```python
from build123d import *

# Parameters (mm, degrees)
BASE_W                                          = 50
BASE_H                                          = 26
BOSS_EXTRUDE2_DEPTH                             = 3
SKETCH2_R                                       = 6.35
BOSS_EXTRUDE1_DEPTH                             = 20
SKETCH7_R                                       = 4.7625
CUT_EXTRUDE1_DEPTH                              = 15
BOSS_EXTRUDE8_REACH                             = 47.531
CSK_FOR_M5_FLAT_HEAD_MACHINE_SCREW2_D           = 5.3
CSK_FOR_M5_FLAT_HEAD_MACHINE_SCREW2_DEPTH       = 10
CSK_FOR_M5_FLAT_HEAD_MACHINE_SCREW2_CSINK_D     = 10.4
CSK_FOR_M5_FLAT_HEAD_MACHINE_SCREW2_CSINK_ANGLE = 90
CSK_FOR_M5_FLAT_HEAD_MACHINE_SCREW2_TIP         = 1.59228064


with BuildPart() as part:
    # Base → Boss-Extrude2 (new body)
    with BuildSketch(Plane.XY):
        Rectangle(BASE_W, BASE_H)
    extrude(amount=BOSS_EXTRUDE2_DEPTH)

    # Sketch6 → Loft2 section 0
    with BuildSketch(Plane.XY.offset(23)):
        with BuildLine():
            Line((-5, 13), (5, 13))
            Line((5, 13), (5, 6.65))
            Line((5, 6.65), (-5, 6.65))
            Line((-5, 6.65), (-5, 13))
        make_face()
    # Sketch5 → Loft2 section 1
    with BuildSketch(Plane.XY.offset(3)):
        with BuildLine():
            Line((-25, 13), (25, 13))
            Line((25, 13), (25, 6.65))
            Line((25, 6.65), (-25, 6.65))
            Line((-25, 6.65), (-25, 13))
        make_face()
    loft()



with BuildPart() as body_2:
    # Sketch2 → Boss-Extrude1 (new body)
    with BuildSketch(Plane(origin=(-16.995934691, 0, 52.308108396), x_dir=(0.9510565162951523, 0, 0.3090169943749514), z_dir=(-0.3090169943749514, 0, 0.9510565162951523))):
        with Locations((11.371412907, 9.08)):
            Circle(SKETCH2_R)
    extrude(amount=-BOSS_EXTRUDE1_DEPTH)

    # Sketch7 → Cut-Extrude1 (cut)
    with BuildSketch(Plane(origin=(-16.995934691, 0, 52.308108396), x_dir=(0.9510565162951523, 0, 0.3090169943749514), z_dir=(-0.3090169943749514, 0, 0.9510565162951523))):
        with Locations((11.371412907, 9.08)):
            Circle(SKETCH7_R)
    extrude(amount=-CUT_EXTRUDE1_DEPTH, mode=Mode.SUBTRACT)


with BuildPart() as part_1:
    add(part.part)

    add(body_2.part)  # Boss-Extrude8 merges body 2
    # Boss-Extrude8: up to this plane
    boss_extrude8_end = Plane(origin=(-0.000738458, 9.08, 36.800937909), z_dir=(-0.3090169943749514, 0, 0.9510565162951523))
    # Sketch17 → Boss-Extrude8 (add, up to the surface)
    with BuildSketch(Plane.XY.offset(23), mode=Mode.PRIVATE) as boss_extrude8_sk1:
        Polygon((-4.751504294, 13.000455244), (-4.751504294, 6.647086382), (4.750367151, 6.647086382), (4.750367151, 13), align=None)
    boss_extrude8_tool1 = split(extrude(boss_extrude8_sk1.sketch, amount=BOSS_EXTRUDE8_REACH, mode=Mode.PRIVATE), bisect_by=boss_extrude8_end, keep=Keep.BOTH, mode=Mode.PRIVATE)
    add(boss_extrude8_tool1.solids().sort_by_distance((-0.000625, 9.823657, 23))[0])

    # CSK for M5 Flat Head Machine Screw2
    with Locations(Plane.XY.offset(3)):
        with Locations((-15, -1.5), (15, -1.5)):
            CounterSinkHole(CSK_FOR_M5_FLAT_HEAD_MACHINE_SCREW2_D / 2, CSK_FOR_M5_FLAT_HEAD_MACHINE_SCREW2_CSINK_D / 2, depth=CSK_FOR_M5_FLAT_HEAD_MACHINE_SCREW2_DEPTH, counter_sink_angle=CSK_FOR_M5_FLAT_HEAD_MACHINE_SCREW2_CSINK_ANGLE)
            with Locations((0, 0, -(CSK_FOR_M5_FLAT_HEAD_MACHINE_SCREW2_DEPTH + CSK_FOR_M5_FLAT_HEAD_MACHINE_SCREW2_TIP / 2))):  # 118° drill point
                Cone(0, CSK_FOR_M5_FLAT_HEAD_MACHINE_SCREW2_D / 2, CSK_FOR_M5_FLAT_HEAD_MACHINE_SCREW2_TIP, mode=Mode.SUBTRACT)


solid = part_1.part
```
Input: part model. Units: mm. Frame: model coordinates. A direction names the side the tool comes from. Coordinates: 2 decimals unless noted, no trailing zeros. Loops run counter-clockwise (first coordinate to the right, second up) from the corner with the lowest first, then second, coordinate; pieces in that order, holes last. Notation, with made-up numbers: M -37,63 L -20,63 A24 cw -20,100 Z; hole C 25,29.5 d3. An arc over 180 degrees is marked long. Use a Markdown table: item, result. Add a question column.
1) Pin query (flat end, axial travel): P1, Ø8, axis at x = 7, z = 27, coming from the +Y side; P2, Ø7, axis at x = 15, y = -1.5, coming from the +Z side; P3, Ø6, axis at x = -11.5, y = -7, coming from the +Z side; P4, Ø4, axis at x = -15, y = -1.5, coming from the +Z side. Return the tip coordinate at first contact, or that it passes through.
2) Section C-C, the plane y = -10. Return the cut outline in (x, z), plus the area to 3 significant figures.
3) Draft query along Z for faces 1 (the conical face through (17.201, -3.188, 0.574)), 2 (the flat face through (-15, 10, 13)), 3 (the flat face through (0, 13, 9)). Return one class per face: +Z half, -Z half, draft (parallel to the pull), parting line (faces both ways), or undercut.
4) Set-up query: faces 4 (the flat face through (4.75, 10, 31)), 5 (the cylindrical face through (-17.528, -0.704, 0.222)), 6 (the flat face through (0, 6.647, 31)), 7 (the flat face through (-7.551, 13.813, 55.377)), 8 (the flat face through (-0.07, 13.96, 36.78)). Return all of +Z, -Z, +X, -X, +Y, -Y with unobstructed straight access to the full face (end or side cutting, diameter ignored); none if empty.
5) Section D-D, the plane y = 11.25. Return the cut outline in (x, z).
6) Line query: L1, parallel to X at y = -1.5, z = 0.35; L2, parallel to Y at x = 15, z = 0.1. Output: solid intervals per line, ascending. Write a range as from..to.
7) Section B-B, the plane z = 28.5. Return the cut outline in (x, y).
8) Section A-A, the plane y = -1.5. Return the cut outline in (x, z).
Answer below:
| question | item | result |
|---|---|---|
| 1 | P1 | y = 13 |
| 1 | P2 | z = 1.3 |
| 1 | P3 | z = 3 |
| 1 | P4 | through |
| 2 | outline | M -25,0 L 25,0 L 25,3 L -25,3 Z |
| 2 | area | 150 mm2 |
| 3 | face 1 | +Z half |
| 3 | face 2 | undercut |
| 3 | face 3 | draft |
| 4 | face 4 | +X, +Y, -Y |
| 4 | face 5 | +Z, -Z |
| 4 | face 6 | +X, -Y |
| 4 | face 7 | +Z, -X, +Y, -Y |
| 4 | face 8 | -Z, +X, +Y |
| 5 | outline | M -25,0 L 25,0 L 25,3 L 5,23 L 4.75,23 L 4.75,38.34 L 5.67,38.65 L -0.51,57.67 L -2.15,57.13 L 2.49,42.87 L -5.58,40.25 L -10.21,54.51 L -11.86,53.98 L -5.68,34.96 L -4.75,35.26 L -4.75,23 L -5,23 L -25,3 Z |
| 6 | L1 | -25..-17.65, -12.35..12.35, 17.65..25 |
| 6 | L2 | -13..-4.15, 1.15..13 |
| 7 | outline | M -4.75,6.65 L 4.75,6.65 L 4.75,13 L -4.75,13 Z |
| 8 | outline | M -25,0 L -17.65,0 L -17.65,0.45 L -20.2,3 L -25,3 Z; M -12.35,0 L 12.35,0 L 12.35,0.45 L 9.8,3 L -9.8,3 L -12.35,0.45 Z; M 17.65,0 L 25,0 L 25,3 L 20.2,3 L 17.65,0.45 Z |
